For this review, use the dimensioned drawing (mm, ordinates from the lowest corner) and the shaded views. A direction names the side the tool comes from. Give positions to 0.01 mm unless a question says otherwise; leave off trailing zeros. Write each loop counter-clockwise with the first axis right and the second up, starting at its lowest first coordinate (ties: lowest second). Pieces come first, ordered by that corner, then holes. Notation, with made-up numbers: M 26.25,39.5 L 76.25,39.5 A25 ccw 76.25,56.5 Z; hole C 32.25,-3 d8. An arc over 180 degrees is marked long. Answer in a Markdown table with one row per item.
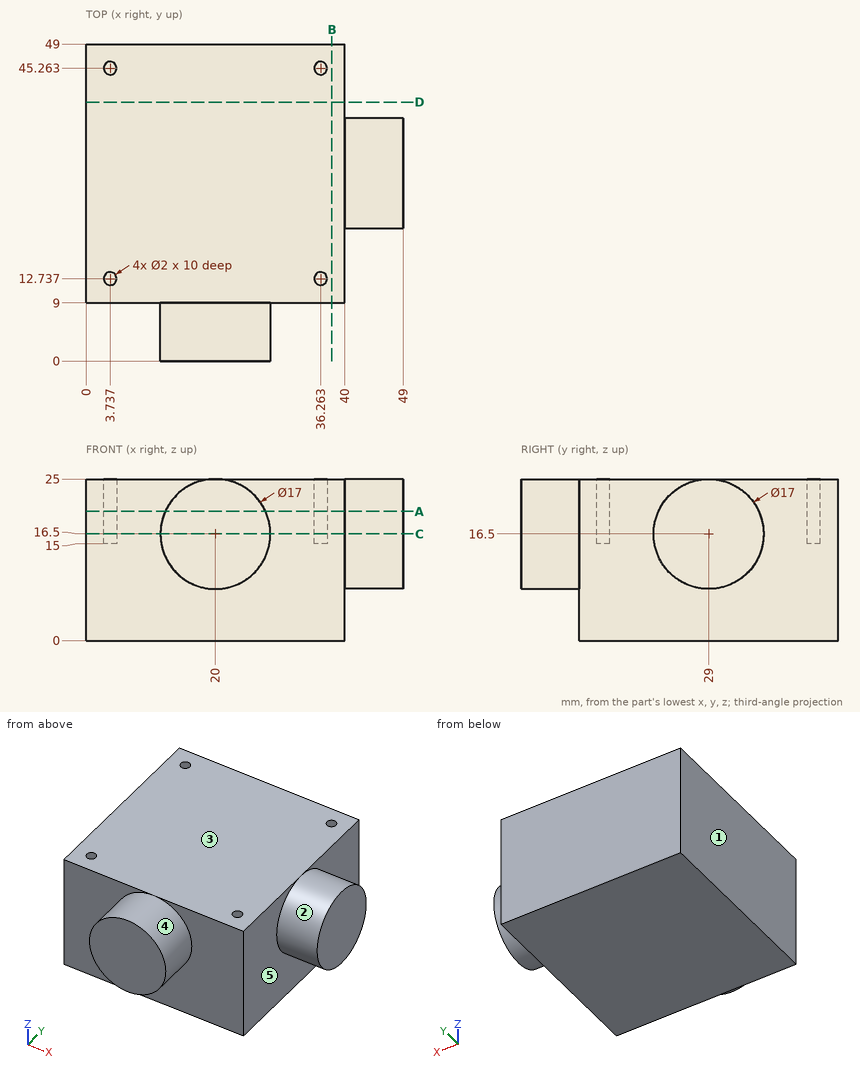
1) Insertion check: P1, Ø1, axis at x = 8, z = 6.5, coming from the -Y side; P2, Ø3, axis at y = 17, z = 11.5, coming from the +X side; P3, Ø0.6, axis at x = 3.5, y = 12.5, coming from the +Z side. Each pin has a flat end and moves straight along its axis. Give the tip position at first contact, or say it passes through.
Geometry says:
| item | result |
|---|---|
| P1 | y = 9 |
| P2 | x = 40 |
| P3 | z = 15 |
2) Add section C-C (z = 16.5). Write out the cut boundary in (x, y), and give its area (3 significant figures).
Geometry says:
| item | result |
|---|---|
| outline | M 0,9 L 11.5,9 L 11.5,0 L 28.5,0 L 28.5,9 L 40,9 L 40,20.5 L 49,20.5 L 49,37.5 L 40,37.5 L 40,49 L 0,49 Z; hole C 3.74,12.74 d2; hole C 3.74,45.26 d2; hole C 36.26,12.74 d2; hole C 36.26,45.26 d2 |
| area | 1,890 mm^2 |
3) The part is to be moulded in two halves that separate along X. For the marked faces 3, 4 and 5, say which applies: released by +X, released by -X, zero draft, split by the parting line, or undercut.
Geometry says:
| item | result |
|---|---|
| face 3 | zero draft |
| face 4 | split by the parting line |
| face 5 | released by +X |
4) Add section D-D (y = 40). Write out the cut boundary in (x, z), and give its area (3 significant figures).
Geometry says:
| item | result |
|---|---|
| outline | M 0,0 L 40,0 L 40,25 L 0,25 Z |
| area | 1,000 mm^2 |
5) Add section A-A (z = 20). Write out the cut boundary in (x, y), and give its area (3 significant figures).
Geometry says:
| item | result |
|---|---|
| outline | M 0,9 L 12.25,9 L 12.25,0 L 27.75,0 L 27.75,9 L 40,9 L 40,21.25 L 49,21.25 L 49,36.75 L 40,36.75 L 40,49 L 0,49 Z; hole C 3.74,12.74 d2; hole C 3.74,45.26 d2; hole C 36.26,12.74 d2; hole C 36.26,45.26 d2 |
| area | 1,870 mm^2 |
6) To check wall thickness, follow probe 1 along Y at (x, z) = (4.5, 22) (1 decimal); probe 2 along X at (y, z) = (22.5, 23.5); probe 3 along Y at (x, z) = (14, 7.5). State the ranges of each line that lie inside material, in increasing order. Write a range as [from, to].
Geometry says:
| item | result |
|---|---|
| probe 1 | [9, 12.1], [13.4, 44.6], [45.9, 49] |
| probe 2 | [0, 40] |
| probe 3 | [9, 49] |
7) For the marked faces 1 and 2, list the 3-axis set-ups (+Z, -Z, +X, -X, +Y, -Y) from which the entire face can be reached by the end or side of a thin tool; tool diameter is ignored.
Geometry says:
| item | result |
|---|---|
| face 1 | +Z, -Z, -X, +Y, -Y |
| face 2 | +X |
8) Add section B-B (x = 38). Write out the cut boundary in (y, z), and give its area (3 significant figures).
Geometry says:
| item | result |
|---|---|
| outline | M 9,0 L 49,0 L 49,25 L 9,25 Z |
| area | 1,000 mm^2 |
